Here's how the part is built. I have some questions about the finished solid (model axes, mm). Round coordinates to 2 decimals unless told otherwise and drop trailing zeros. Loops run counter-clockwise (first coordinate to the right, second up) from the corner with the lowest first, then second, coordinate; pieces in that order, holes last. Notation, with made-up numbers: M -35,46.5 L -26,46.5 A15 cw -26,50.5 Z; hole C -20,32.5 d3. An arc over 180 degrees is marked long. Answer as a JSON object with one key per item and string values.
from build123d import *

# Parameters (mm, degrees)
F0_R     = 2
F0_R_2   = 1.15
F1_DEPTH = 8
F3_R     = 2.5
F3_R_2   = 2
F4_DEPTH = 4


# Not quite as in the source:
# - a fillet or chamfer that OpenCascade refuses, or shapes differently, is made with other operations: its cross-section is extruded or revolved along the edge and cut away or added


with BuildPart() as f1:
    # F0 (on Top) → F1 (new body)
    with BuildSketch(Plane.XY):
        Circle(F0_R)
        Circle(F0_R_2, mode=Mode.SUBTRACT)
    extrude(amount=F1_DEPTH)

    # F3 (on offset) → F4 (join, through all)
    with BuildSketch(Plane.XY.offset(4)):
        Circle(F3_R)
        Circle(F3_R_2, mode=Mode.SUBTRACT)
    extrude(amount=F4_DEPTH)

    # F5: fillet of radius 2 on 1 edges, made by hand

    # F5_s1 → F5_t2 (revolve, cut)
    with BuildSketch(Plane.XZ):
        with BuildLine():
            ThreePointArc((2.5, 6.1085719681), (2.1278820596, 7.2704669719), (1.15, 8))
            Line((1.15, 8), (2.5, 8))
            Line((2.5, 8), (2.5, 6.1085719681))
        make_face()
    revolve(axis=Axis((0, 0, 8), (0, 0, 1)), mode=Mode.SUBTRACT)


solid = f1.part
Item 1: I'm going to push a flat-ended pin straight in: pin 1 Ø1.5 at (x, z) = (1, 2.5) entering from +Y. Where does the tip first touch, or does it pass through?
Resolved:
{"pin 1": "y = 1.98"}
Item 2: Please list where these lines run through material, in increasing order: probe 1 along Y at (x, z) = (0, 3.5); probe 2 along Y at (x, z) = (0, 6); probe 3 along X at (y, z) = (0.45, 6.75). Write a range as from..to.
Resolved:
{"probe 1": "-2..-1.15, 1.15..2", "probe 2": "-2.5..-1.15, 1.15..2.5", "probe 3": "-2.35..-1.06, 1.06..2.35"}
Item 3: If we mould it in two halves opening along Y, with no side actions, what happens to faces 1 (the face through (-0.91, -0.7, 3.94)), 2 (the face through (-1, 2, 4)), 3 (the face through (0, -2, 2))? For each: pulls with the +Y half, pulls with the -Y half, needs draft (parallel to the pull), parting line crosses it, or undercut.
Resolved:
{"face 1": "undercut", "face 2": "needs draft", "face 3": "parting line crosses it"}
Item 4: I want a section at B-B, the plane z = 4.25. Please give me the cut outline in (x, y), then the cut area to 3 significant figures.
Resolved:
{"outline": "C 0,0 d5; hole C 0,0 d2.3", "area": "15.5 mm²"}
Item 5: I want a section at A-A, the plane z = 0.5. Please give me the cut outline in (x, y), then the cut area to 3 significant figures.
Resolved:
{"outline": "C 0,0 d4; hole C 0,0 d2.3", "area": "8.41 mm²"}
